```python
from build123d import *

# Parameters (mm, degrees)
BOSS_EXTRUDE1_DEPTH = 3
SKETCH2_R           = 1.5
CUT_EXTRUDE1_DEPTH  = 3
SKETCH3_R           = 30
SKETCH3_R_2         = 15
CUT_EXTRUDE2_DEPTH  = 3


with BuildPart() as part:
    # Sketch1 → Boss-Extrude1 (new body)
    with BuildSketch(Plane.XY):
        with BuildLine():
            Line((-32.133468612, 81.630943295), (32.133468612, 81.630943295))
            Line((32.133468612, 81.630943295), (81.630943295, 32.133468612))
            Line((81.630943295, 32.133468612), (81.630943295, -32.133468612))
            Line((81.630943295, -32.133468612), (32.133468612, -81.630943295))
            add(Edge.make_bspline(
                [(-32.133468612, -81.630943295), (-26.315604905, -78.929469601), (-17.458466972, -75.90692924), (-6.459846686, -74.366971031), (0.503945588, -74.095540146), (13.381410653, -74.737409183), (24.194527132, -77.919288079), (32.133468612, -81.630943295)],
                knots=[0, 0, 0, 0, 0.289771888, 0.418866631, 0.500125988, 0.604148798, 1, 1, 1, 1], degree=3))
            Line((-32.133468612, -81.630943295), (-81.630943295, -32.133468612))
            Line((-81.630943295, -32.133468612), (-81.630943295, 32.133468612))
            Line((-81.630943295, 32.133468612), (-32.133468612, 81.630943295))
        make_face()
    extrude(amount=BOSS_EXTRUDE1_DEPTH)

    # Sketch2 → Cut-Extrude1 (cut)
    with BuildSketch(Plane.XY.offset(3)):
        with Locations((-39.204536424, -39.204536424)):
            Circle(SKETCH2_R)
        with Locations((39.204536424, -39.204536424)):
            Circle(SKETCH2_R)
        with Locations((39.204536424, 39.204536424)):
            Circle(SKETCH2_R)
        with Locations((-39.204536424, 39.204536424)):
            Circle(SKETCH2_R)
    extrude(amount=-CUT_EXTRUDE1_DEPTH, mode=Mode.SUBTRACT)

    # Sketch3 → Cut-Extrude2 (cut)
    with BuildSketch(Plane.XY.offset(3)):
        Circle(SKETCH3_R)
        with Locations((0, 30)):
            Circle(SKETCH3_R_2)
        with Locations((0, -30)):
            Circle(SKETCH3_R_2)
        with Locations((30, 0)):
            Circle(SKETCH3_R_2)
        with Locations((-30, 0)):
            Circle(SKETCH3_R_2)
    extrude(amount=-CUT_EXTRUDE2_DEPTH, mode=Mode.SUBTRACT)


solid = part.part
```
Geometry check sheet. Reference: the model listing, model coordinates, mm. A direction names the side the tool comes from. Coordinates: 2 decimals unless noted, no trailing zeros. Write each loop counter-clockwise with the first axis right and the second up, starting at its lowest first coordinate (ties: lowest second). Pieces come first, ordered by that corner, then holes. Notation, with made-up numbers: M -1.5,-25.75 L 29.5,-25.75 A17 cw 29.5,3.25 Z; hole C -34,58.5 d6. An arc over 180 degrees is marked long. Answer as a JSON object with one key per item and string values.
1. Scan lines: L1, parallel to Y at x = -39, z = 0.65; L2, parallel to X at y = 30, z = 2.1; L3, parallel to X at y = -28, z = 0.75. Record each from-to range of solid material in increasing order.
Answers below:
{"L1": "y = -74.76 to -40.69, -37.72 to -12, 12 to 37.72, 40.69 to 74.76", "L2": "x = -81.63 to -15, 15 to 81.63", "L3": "x = -81.63 to -14.87, 14.87 to 81.63"}
2. Section check D-D, the plane x = 64.5. Enter the section's corners in (y, z), plus the area to 3 significant figures.
Answers below:
{"outline": "M -49.26,0 L 49.26,0 L 49.26,3 L -49.26,3 Z", "area": "296 mm²"}
3. Section check C-C, the plane z = 1. Give the number of separate pieces and of enclosed holes in the cut face, plus the area to 3 significant figures.
Answers below:
{"separate pieces": "1", "enclosed holes": "5", "area": "17,000 mm²"}
4. Section check A-A, the plane y = 0. Enter the section's corners in (x, z).
Answers below:
{"outline": "M -81.63,0 L -45,0 L -45,3 L -81.63,3 Z; M 45,0 L 81.63,0 L 81.63,3 L 45,3 Z"}
5. Draft check along X on faces 3 (the flat face through (-57.229, 56.536, 1.479)), 4 (the cylindrical face through (-45, 0, 2)), 5 (the cylindrical face through (21.296, 21.13, 1.521)), 6 (the flat face through (57.229, -56.536, 1.479)). Enter one of: released by +X, released by -X, zero draft, split by the parting line, or undercut.
Answers below:
{"face 3": "released by -X", "face 4": "undercut", "face 5": "undercut", "face 6": "released by +X"}
6. Tool access check on faces 1 (the cylindrical face through (-21.296, -21.13, 1.521)), 2 (the flat face through (-56.536, -57.229, 1.479)). Record the directions out of +Z, -Z, +X, -X, +Y, -Y that give a thin tool (end or side, any length) a straight path to the whole face; none if there is none.
Answers below:
{"face 1": "+Z, -Z", "face 2": "+Z, -Z, -X, -Y"}
7. Section check B-B, the plane y = -30. Enter the section's corners in (x, z).
Answers below:
{"outline": "M -81.63,0 L -15,0 L -15,3 L -81.63,3 Z; M 15,0 L 81.63,0 L 81.63,3 L 15,3 Z"}
8. Go/stop test with a flat-tipped pin: pin 1 Ø2.5 at (x, y) = (39.2, -39.2) entering from +Z. Record where the tip stops, or that it passes through.
Answers below:
{"pin 1": "passes through"}
